For this review, take the finished solid that the model builds, in its own axes (mm). A direction names the side the tool comes from. Give positions to 0.01 mm unless a question says otherwise; leave off trailing zeros. Write each loop counter-clockwise with the first axis right and the second up, starting at its lowest first coordinate (ties: lowest second). Pieces come first, ordered by that corner, then holes. Notation, with made-up numbers: (4.5, -34.5) -> (23.5, -34.5) arc R15 cw to (23.5, -27.5) -> close; hole circle Ø2 at (-2.5, 51.5). An arc over 180 degrees is marked (long way). Return JSON: item names as keys, results as strings.
from build123d import *

# Parameters (mm, degrees)
FILLET1_R = 1
SKETCH3_W = 0.8
SKETCH3_H = 8.5


with BuildPart() as part:
    # Sketch1 → Revolve1 (revolve)
    with BuildSketch(Plane.XY):
        Polygon((-8.5, -48), (-8.5, -19.8), (-9.5, -19.8), (-9.5, 0), (-10, 0), (-10, 1.5), (-8.5, 1.5), (-8.5, 13.5), (-10, 13.5), (-10, 15), (0, 15), (0, -34), (-4, -34), (-4, -48), align=None)
    revolve(axis=Axis((0, 15, 0), (0, -1, 0)))

    # Fillet1
    fillet1_edges = [part.edges().sort_by_distance(p)[0] for p in [
        (8.5, -48, 0),
        (4, -48, 0),
    ]]
    fillet(fillet1_edges, radius=FILLET1_R)

    # Sketch3 → M2x0.4 Tapped Hole1 (revolve, cut)
    with BuildSketch(Plane(origin=(0, -40, 0), x_dir=(0, 1, 0), z_dir=(1, 0, 0))):
        with Locations((0.4, 4.25)):
            Rectangle(SKETCH3_W, SKETCH3_H)
    revolve(axis=Axis((0, -40, -6.35), (0, 0, 1)), mode=Mode.SUBTRACT)


solid = part.part
1. Add section C-C, the plane y = -36. State the section outline as (x, z) points, plus the area to 3 significant figures.
Results found:
{"outline": "circle Ø17 at (0, 0); hole circle Ø8 at (0, 0)", "area": "177 mm²"}
2. For pin 1 (1.3 mm diameter, centred on x = 0, y = -40, fed in from +Z); pin 2 (3 mm diameter, centred on y = 2, z = 1, fed in from -X); pin 3 (10 mm diameter, centred on x = 3, y = -12, fed in from +Z); pin 4 (10 mm diameter, centred on x = -1, y = -28.5, fed in from +Z), all flat-tipped, find the tip position at first contact; note any pin that passes through.
Results found:
{"pin 1": "stops at z = -3.95", "pin 2": "stops at x = -10", "pin 3": "stops at z = 9.5", "pin 4": "stops at z = 8.5"}
3. The part is to be moulded in two halves that separate along X. For faces 1 (the cylindrical face through (-4.57, 7.584, -7.167)), 2 (the flat face through (-4.5, 13.5, 7.4)), 3 (the flat face through (0, -34, 0)), say which applies: +X half, -X half, draft (parallel to the pull), parting line (faces both ways), or undercut.
Results found:
{"face 1": "parting line", "face 2": "draft", "face 3": "undercut"}
4. To check wall thickness, follow probe 1 along Y at (x, z) = (7.5, 6.5); probe 2 along Z at (x, y) = (0, -43). State the ranges of each line that lie inside material, in increasing order.
Results found:
{"probe 1": "y = 0 to 1.5, 13.5 to 15", "probe 2": "z = -8.5 to -4, 4 to 8.5"}
5. Add section B-B, the plane z = 0. State the section outline as (x, y) points, plus the area to 3 significant figures.
Results found:
{"outline": "(-10, 0) -> (-9.5, 0) -> (-9.5, -19.8) -> (-8.5, -19.8) -> (-8.5, -47) arc R1 ccw to (-7.5, -48) -> (-5, -48) arc R1 ccw to (-4, -47) -> (-4, -34) -> (4, -34) -> (4, -47) arc R1 ccw to (5, -48) -> (7.5, -48) arc R1 ccw to (8.5, -47) -> (8.5, -19.8) -> (9.5, -19.8) -> (9.5, 0) -> (10, 0) -> (10, 1.5) -> (8.5, 1.5) -> (8.5, 13.5) -> (10, 13.5) -> (10, 15) -> (-10, 15) -> (-10, 13.5) -> (-8.5, 13.5) -> (-8.5, 1.5) -> (-10, 1.5) -> close", "area": "1,010 mm²"}
6. For faces 4 (the flat face through (-2.2, -19.8, 8.4)), 5 (the cylindrical face through (-0.24, -39.237, 6.242)), 6 (the flat face through (4.5, 1.5, 7.4)), list the 3-axis set-ups (+Z, -Z, +X, -X, +Y, -Y) from which the entire face can be reached by the end or side of a thin tool; tool diameter is ignored.
Results found:
{"face 4": "-Y", "face 5": "+Z", "face 6": "none"}
